Could you check a few things on this model? Use its own coordinates, in mm. A direction names the side the tool comes from. Coordinates: 2 decimals unless noted, no trailing zeros. Loops run counter-clockwise (first coordinate to the right, second up) from the corner with the lowest first, then second, coordinate; pieces in that order, holes last. Notation, with made-up numbers: (59, 56) -> (82, 56) arc R7 ccw to (82, 67) -> close; hole circle Ø8 at (2.25, 1.25). An arc over 180 degrees is marked (long way). One line per question, with ' | ' between items.
```python
from build123d import *

# Parameters (mm, degrees)
BOSS_EXTRUDE1_DEPTH = 10


with BuildPart() as part:
    # Sketch1 → Boss-Extrude1 (new body)
    with BuildSketch(Plane.XY.offset(232.248004761)):
        Polygon((-82.257473883, 116.914823413), (-82.257473883, 82.464823413), (-82.257473883, 72.464823413), (-52.257473883, 72.464823413), (-52.257473883, 82.464823413), (-29.482473883, 82.464823413), (-29.482473883, 116.914823413), (14.967526117, 116.914823413), (14.967526117, 82.464823413), (37.742526117, 82.464823413), (37.742526117, 72.464823413), (67.742526117, 72.464823413), (67.742526117, 82.464823413), (67.742526117, 116.914823413), (37.52195778, 116.914823413), (37.52195778, 126.914823413), (-52.036905545, 126.914823413), (-52.036905545, 116.914823413), align=None)
    extrude(amount=-BOSS_EXTRUDE1_DEPTH)


solid = part.part
```
Q1. We'd pull the mould along X, two halves only. Please class faces 5 (the face through (-7, 126.915, 227)), 6 (the face through (67.743, 94, 227)), 7 (the face through (-82.257, 95, 227)), 8 (the face through (14.968, 100, 227)): released by +X, released by -X, zero draft, split by the parting line, or undercut.
Values follow:
face 5: zero draft | face 6: released by +X | face 7: released by -X | face 8: undercut
Q2. Imagine slicing it at C-C on y = 77. Write out the boundary of the cut face in (x, z).
Values follow:
outline: (-82.26, 222.25) -> (-52.26, 222.25) -> (-52.26, 232.25) -> (-82.26, 232.25) -> close; (37.74, 222.25) -> (67.74, 222.25) -> (67.74, 232.25) -> (37.74, 232.25) -> close
Q3. Imagine slicing it at D-D on x = 12.5. Write out the boundary of the cut face in (y, z), plus the area to 3 significant figures.
Values follow:
outline: (116.91, 222.25) -> (126.91, 222.25) -> (126.91, 232.25) -> (116.91, 232.25) -> close | area: 100 mm2
Q4. Imagine slicing it at A-A on y = 88.5. Write out the boundary of the cut face in (x, z), plus the area to 3 significant figures.
Values follow:
outline: (-82.26, 222.25) -> (-29.48, 222.25) -> (-29.48, 232.25) -> (-82.26, 232.25) -> close; (14.97, 222.25) -> (67.74, 222.25) -> (67.74, 232.25) -> (14.97, 232.25) -> close | area: 1,060 mm2
Q5. For faces 1 (the face through (53, 116.915, 227)), 2 (the face through (-67, 72.465, 227)), 3 (the face through (-67, 116.915, 227)), 4 (the face through (-8, 116.915, 227)), which set-ups out of +Z, -Z, +X, -X, +Y, -Y let a thin tool reach every point of the face, with its end or its side?
Values follow:
face 1: +Z, -Z, +X, +Y | face 2: +Z, -Z, +X, -X, -Y | face 3: +Z, -Z, -X, +Y | face 4: +Z, -Z, -Y
Q6. For pin 1 (5 mm diameter, centred on x = 28, z = 228, fed in from -Y); pin 2 (3 mm diameter, centred on x = -17, z = 228, fed in from -Y); pin 3 (5 mm diameter, centred on x = 46, z = 226, fed in from +Y), each with a flat end and sliding along its axis, tell me the tip position at first contact or that it passes through.
Values follow:
pin 1: stops at y = 82.46 | pin 2: stops at y = 116.91 | pin 3: stops at y = 116.91
Q7. Please list where these lines run through material, in increasing order: L1, parallel to X at y = 76, z = 229; L2, parallel to X at y = 86, z = 229.25; L3, parallel to Y at x = -65, z = 227. Write a range as [from, to].
Values follow:
L1: x = [-82.26, -52.26], [37.74, 67.74] | L2: x = [-82.26, -29.48], [14.97, 67.74] | L3: y = [72.46, 116.91]
Q8. Imagine slicing it at B-B on z = 228.5. Write out the boundary of the cut face in (x, y).
Values follow:
outline: (-82.26, 72.46) -> (-52.26, 72.46) -> (-52.26, 82.46) -> (-29.48, 82.46) -> (-29.48, 116.91) -> (14.97, 116.91) -> (14.97, 82.46) -> (37.74, 82.46) -> (37.74, 72.46) -> (67.74, 72.46) -> (67.74, 116.91) -> (37.52, 116.91) -> (37.52, 126.91) -> (-52.04, 126.91) -> (-52.04, 116.91) -> (-82.26, 116.91) -> close
